Here's how the part is built. I have some questions about the finished solid (model axes, mm). A direction names the side the tool comes from. Coordinates: 2 decimals unless noted, no trailing zeros. Write each loop counter-clockwise with the first axis right and the second up, starting at its lowest first coordinate (ties: lowest second). Pieces come first, ordered by that corner, then holes. Notation, with made-up numbers: (-30.5, 7) -> (-21.5, 7) arc R24 cw to (-21.5, 35) -> close; hole circle Ø3 at (64.25, 19). An arc over 180 degrees is marked (long way). Put each result on its own line as item: value. Start each with the question number.
Item 1: For pin 1 (2.5 mm diameter, centred on y = 0, z = 28, fed in from +X); pin 2 (1.1 mm diameter, centred on x = -0.5, z = 2.5, fed in from -Y); pin 3 (3 mm diameter, centred on x = -0.5, z = 5, fed in from +Y), each with a flat end and sliding along its axis, tell me the tip position at first contact or that it passes through.
Item 2: I want a section at C-C, the plane y = 2.25. List the corners of the cut face in (x, z) for me, then the cut area to 3 significant figures.
Item 3: I need wall thicknesses on line 1 (X direction, y = 0, z = 13) (3 decimals); line 2 (X direction, y = -0.5, z = 10.5); line 3 (Z direction, x = 0, y = 1.25). Which ranges of each line are inside material? Lowest first, please. Write a range as [from, to].
Item 4: On a 3-axis mill with a long thin cutter (end or side, diameter ignored), from which of +Z, -Z, +X, -X, +Y, -Y can I reach the whole of each face in a straight line? I mean faces 4 (the face through (1.4, 2.6, 6.5)), 5 (the face through (-1.32, 2.34, 21.29)), 6 (the face through (-1.4, -2.6, 6.5)), 7 (the face through (1.4, -2.6, 6.5)), 8 (the face through (2.685, 0, 21)). Say none if no direction works.
Item 5: If we mould it in two halves opening along X, with no side actions, what happens to faces 1 (the face through (0, -3.05, 3)), 2 (the face through (1.32, -2.34, 21.29)), 3 (the face through (0, 0, 35))? For each: released by +X, released by -X, zero draft, split by the parting line, or undercut.
Item 6: I want a section at A-A, the plane z = 22.5. List the corners of the cut face in (x, y) for me (3 decimals).
Item 7: I want a section at B-B, the plane x = 0.5. List the corners of the cut face in (y, z) for me, then the cut area to 3 significant figures.
Item 8: I want a section at D-D, the plane z = 3. List the corners of the cut face in (x, y) for me (3 decimals), then the cut area to 3 significant figures.
from build123d import *

# Parameters (mm, degrees)
F1_DEPTH = 6.5
F3_DEPTH = 30
F4_R     = 1.625
F5_DEPTH = 35


with BuildPart() as f1:
    # F0 (on Top) → F1 (new body)
    with BuildSketch(Plane.XY):
        Polygon((-3.521837, 0), (-1.760918, -3.05), (1.760918, -3.05), (3.521837, 0), (1.760918, 3.05), (-1.760918, 3.05), align=None)
    extrude(amount=F1_DEPTH)

    # F2 (on face) → F3 (join)
    with BuildSketch(Plane.XY.offset(6.5)):
        Polygon((2.684679, 1.55), (0, 3.1), (-2.684679, 1.55), (-2.684679, -1.55), (0, -3.1), (2.684679, -1.55), align=None)
    extrude(amount=F3_DEPTH)

    # F4 (on face) → F5 (cut)
    with BuildSketch(Plane(origin=(0, 0, 0), x_dir=(1, 0, 0), z_dir=(0, 0, -1))):
        Circle(F4_R)
    extrude(amount=-F5_DEPTH, mode=Mode.SUBTRACT)


solid = f1.part
Calculated:
1. pin 1: stops at x = 2.68
1. pin 2: stops at y = -3.05
1. pin 3: stops at y = 3.05
2. outline: (-2.22, 0) -> (2.22, 0) -> (2.22, 6.5) -> (1.47, 6.5) -> (1.47, 36.5) -> (-1.47, 36.5) -> (-1.47, 6.5) -> (-2.22, 6.5) -> close
2. area: 117 mm2
3. line 1: x = [-2.685, -1.625], [1.625, 2.685]
3. line 2: x = [-2.68, -1.55], [1.55, 2.68]
3. line 3: z = [35, 36.5]
4. face 4: +Z, +X, +Y
4. face 5: +Z, -X, +Y
4. face 6: +Z, -X, -Y
4. face 7: +Z, +X, -Y
4. face 8: +Z, +X, +Y, -Y
5. face 1: zero draft
5. face 2: released by +X
5. face 3: undercut
6. outline: (-2.685, -1.55) -> (0, -3.1) -> (2.685, -1.55) -> (2.685, 1.55) -> (0, 3.1) -> (-2.685, 1.55) -> close; hole circle Ø3.25 at (0, 0)
7. outline: (-3.05, 0) -> (-1.55, 0) -> (-1.55, 35) -> (1.55, 35) -> (1.55, 0) -> (3.05, 0) -> (3.05, 6.5) -> (2.81, 6.5) -> (2.81, 36.5) -> (-2.81, 36.5) -> (-2.81, 6.5) -> (-3.05, 6.5) -> close
7. area: 100 mm2
8. outline: (-3.522, 0) -> (-1.761, -3.05) -> (1.761, -3.05) -> (3.522, 0) -> (1.761, 3.05) -> (-1.761, 3.05) -> close; hole circle Ø3.25 at (0, 0)
8. area: 23.9 mm2
